Geometry: final body of the model. Coordinates: model frame, mm. A direction names the side the tool comes from. Give positions to 0.01 mm unless a question says otherwise; leave off trailing zeros. Order: outer loops, then holes, each group sorted by start corner. A loop starts at its lowest first (then second) coordinate and runs counter-clockwise, first axis right, second up. Notation, with made-up numbers: (-22, -37) - (31, -37) arc R12 cw to (31, -16) - close; hole circle Ø2 at (-7, -1.75). An arc over 180 degrees is marked (long way). Use one line per item in the form item = value.
from build123d import *

# Parameters (mm, degrees)
BOSS_EXTRUDE1_DEPTH = 10
SKETCH3_W           = 30
SKETCH3_H           = 34.126910457
BOSS_EXTRUDE2_DEPTH = 8
FILLET1_R           = 1
SKETCH5_R           = 2
CUT_EXTRUDE2_DEPTH  = 63.999765085
SKETCH6_R           = 13.65
CUT_EXTRUDE3_DEPTH  = 8


with BuildPart() as part:
    # Sketch2 → Boss-Extrude1 (new body)
    with BuildSketch(Plane.XY):
        with BuildLine():
            Line((22.912878475, 16.112283523), (-17.087121525, 16.112283523))
            Line((-17.087121525, 16.112283523), (-17.087121525, -17.887716477))
            Line((-17.087121525, -17.887716477), (22.912878475, -17.887716477))
            ThreePointArc((22.912878475, -17.887716477), (39.912878475, -0.887716477), (22.912878475, 16.112283523))
        make_face()
    extrude(amount=BOSS_EXTRUDE1_DEPTH)

    # Sketch3 → Boss-Extrude2 (add)
    with BuildSketch(Plane.ZY.offset(17.087121525)):
        with Locations((5, -0.824261249)):
            Rectangle(SKETCH3_W, SKETCH3_H)
    extrude(amount=-BOSS_EXTRUDE2_DEPTH)

    # Fillet1
    fillet1_edges = [part.edges().sort_by_distance(p)[0] for p in [
        (-9.087121525, -0.887716477, 0),
        (-9.087121525, -0.887716477, 10),
    ]]
    fillet(fillet1_edges, radius=FILLET1_R)

    # Sketch5 → Cut-Extrude2 (cut, through all)
    with BuildSketch(Plane.ZY.offset(17.087121525)):
        with Locations(Location((-5, -0.824261249, 0), (0, 0, 270))):
            Circle(SKETCH5_R)
        with Locations(Location((15, -0.824261249, 0), (0, 0, 270))):
            Circle(SKETCH5_R)
    extrude(amount=-CUT_EXTRUDE2_DEPTH, mode=Mode.SUBTRACT)

    # Sketch6 → Cut-Extrude3 (cut)
    with BuildSketch(Plane(origin=(0, 0, 0), x_dir=(-1, 0, 0), z_dir=(0, 0, -1))):
        with Locations((-22.912878475, -0.887716477)):
            Circle(SKETCH6_R)
    extrude(amount=-CUT_EXTRUDE3_DEPTH, mode=Mode.SUBTRACT)


solid = part.part
(1) Cut plane A-A on z = 15. Output: boundary loops of the cut face in (x, y).
Computed values:
outline = (-17.09, -17.89) - (-9.09, -17.89) - (-9.09, -2.82) - (-17.09, -2.82) - close; (-17.09, 1.18) - (-9.09, 1.18) - (-9.09, 16.24) - (-17.09, 16.24) - close
(2) Contact query for flat-ended pins moving along their axis: pin 1 Ø10 at (x, z) = (-0.5, 16.5) entering from -Y; pin 2 Ø16.5 at (x, y) = (22.91, -0.89) entering from -Z; pin 3 Ø6 at (x, z) = (12.5, 8) entering from +Y; pin 4 Ø6.5 at (y, z) = (-0.82, -5) entering from +X. Output: stop coordinate, or through.
Computed values:
pin_1 = through
pin_2 = 8
pin_3 = 16.11
pin_4 = -9.09
(3) Cut plane C-C on y = -8.5. Output: boundary loops of the cut face in (x, z), plus the area to 3 significant figures.
Computed values:
outline = (-17.09, -10) - (-9.09, -10) - (-9.09, -1) arc R1 cw to (-8.09, 0) - (11.58, 0) - (11.58, 8) - (34.24, 8) - (34.24, 0) - (38.11, 0) - (38.11, 10) - (-8.09, 10) arc R1 cw to (-9.09, 11) - (-9.09, 20) - (-17.09, 20) - close
area = 531 mm²
(4) Ray query, line 1 along Z through (x, y) = (-11, -2); line 2 along Z through (x, y) = (9, 9.5); line 3 along X through (y, z) = (-12, -5.25). Return the intervals inside material, ascending.
Computed values:
line_1 = -10 to -6.62, -3.38 to 13.38, 16.62 to 20
line_2 = 0 to 10
line_3 = -17.09 to -9.09
(5) Reachability of faces 4 (the face through (10.304, -6.116, 3.944)), 5 (the face through (16, -1, 10)), 6 (the face through (5, -1, 0)), 7 (the face through (7, 16.112, 5)) from +Z, -Z, +X, -X, +Y, -Y: full face, straight path, thin tool, end or side. Return the list, or none.
Computed values:
face_4 = -Z
face_5 = +Z, +X, +Y, -Y
face_6 = -Z, +X, +Y, -Y
face_7 = +Z, -Z, +X, +Y
(6) Cut plane B-B on x = -12. Output: boundary loops of the cut face in (y, z).
Computed values:
outline = (-17.89, -10) - (16.24, -10) - (16.24, 20) - (-17.89, 20) - close; hole circle Ø4 at (-0.82, -5); hole circle Ø4 at (-0.82, 15)
(7) Pull-direction query (Z, two-part tool) for faces 1 (the face through (-13.143, -0.564, 16.983)), 2 (the face through (23, -1, 8)), 3 (the face through (39.91, -1.26, 4.93)); classes: released by +Z, released by -Z, zero draft, split by the parting line, or undercut.
Computed values:
face_1 = undercut
face_2 = released by -Z
face_3 = zero draft
(8) Cut plane D-D on x = 33.5. Output: boundary loops of the cut face in (y, z).
Computed values:
outline = (-14.19, 0) - (-9.5, 0) - (-9.5, 8) - (7.73, 8) - (7.73, 0) - (12.41, 0) - (12.41, 10) - (-14.19, 10) - close
